```python
from build123d import *

# Parameters (mm, degrees)
BOSS_EXTRUDE1_DEPTH      = 3.302
BOSS_EXTRUDE1_DEPTH_BACK = 17.018
SKETCH2_W                = 11.43
SKETCH2_H                = 12.7
SKETCH2_5_W              = 5.136925293
SKETCH2_5_H              = 12.7
SKETCH2_5_R              = 1.905
BOSS_EXTRUDE2_DEPTH      = 2.54
BOSS_EXTRUDE3_DEPTH      = 2.54
SKETCH4_R                = 2.286
BOSS_EXTRUDE4_DEPTH      = 5.08


with BuildPart() as part:
    # Sketch2 → Boss-Extrude1 (new, two sides: drawn at the far end of the back side and taken through both)
    with BuildSketch(Plane.XY.offset(-BOSS_EXTRUDE1_DEPTH_BACK)):
        with Locations((-75.585738581, 60.932338755)):
            Rectangle(SKETCH2_W, SKETCH2_H)
        with Locations((-87.015738581, 60.932338755)):
            Rectangle(SKETCH2_W, SKETCH2_H)
    extrude(amount=BOSS_EXTRUDE1_DEPTH + BOSS_EXTRUDE1_DEPTH_BACK)

    # Sketch2_5 → Boss-Extrude2 (add)
    # profile 1 of 2: a face of its own
    with BuildSketch(Plane.XY):
        with Locations((-67.302275935, 60.932338755)):
            Rectangle(SKETCH2_5_W, SKETCH2_5_H)
        with Locations((-67.120738581, 60.932338755)):
            Circle(SKETCH2_5_R, mode=Mode.SUBTRACT)
    # profile 2 of 2: a face of its own
    with BuildSketch(Plane.XY):
        with Locations((-95.299201228, 60.932338755)):
            Rectangle(SKETCH2_5_W, SKETCH2_5_H)
        with Locations((-95.480738581, 60.932338755)):
            Circle(SKETCH2_5_R, mode=Mode.SUBTRACT)
    extrude(amount=-BOSS_EXTRUDE2_DEPTH)

    # Sketch3 → Boss-Extrude3 (add)
    with BuildSketch(Plane.XY.offset(3.302)):
        with BuildLine():
            ThreePointArc((-81.923038581, 63.525721047), (-92.730738581, 60.932338755), (-81.923038581, 58.338956464))
            ThreePointArc((-81.923038581, 58.338956464), (-78.633738581, 60.932338755), (-81.923038581, 63.525721047))
        make_face()
    extrude(amount=BOSS_EXTRUDE3_DEPTH)

    # Sketch4 → Boss-Extrude4 (add)
    with BuildSketch(Plane.XY.offset(5.842)):
        with Locations((-87.015738581, 60.932338755)):
            Circle(SKETCH4_R)
    extrude(amount=BOSS_EXTRUDE4_DEPTH)


solid = part.part
```
Here's how the part is built. I have some questions about the finished solid (model axes, mm). A direction names the side the tool comes from. Round coordinates to 2 decimals unless told otherwise and drop trailing zeros. Order: outer loops, then holes, each group sorted by start corner. A loop starts at its lowest first (then second) coordinate and runs counter-clockwise, first axis right, second up. Notation, with made-up numbers: M 11.25,-22 L 53.25,-22 A23 ccw 53.25,5 Z; hole C -28,-4.75 d8. An arc over 180 degrees is marked long. Answer in a Markdown table with one row per item.
Item 1: For faces 1 (the face through (-92.731, 61, -10)), 2 (the face through (-92.731, 61, 2)), 3 (the face through (-69, 62, -2.54)), 4 (the face through (-92.727, 61.146, 4.554)), 5 (the face through (-69, 62, 0)), which set-ups out of +Z, -Z, +X, -X, +Y, -Y let a thin tool reach every point of the face, with its end or its side?
A:
| item | result |
|---|---|
| face 1 | -Z, -X, +Y, -Y |
| face 2 | +Z, -X, +Y, -Y |
| face 3 | -Z, +X, +Y, -Y |
| face 4 | +Z |
| face 5 | +Z, +X, +Y, -Y |
Item 2: I'm going to push flat-ended pins straight in: pin 1 (5.5 mm diameter, centred on x = -82, y = 60, fed in from +Z); pin 2 (2.5 mm diameter, centred on y = 59, z = 2.5, fed in from -X); pin 3 (5.5 mm diameter, centred on x = -67.5, y = 60.5, fed in from +Z); pin 4 (3 mm diameter, centred on x = -67.12, y = 60.93, fed in from -Z). Where does each tip first touch, or does it pass through?
A:
| item | result |
|---|---|
| pin 1 | stops at z = 5.84 |
| pin 2 | stops at x = -92.73 |
| pin 3 | stops at z = 3.3 |
| pin 4 | passes through |
Item 3: Imagine slicing it at D-D, the plane y = 64.5. Write out the boundary of the cut face in (x, z).
A:
| item | result |
|---|---|
| outline | M -97.87,-2.54 L -92.73,-2.54 L -92.73,-17.02 L -69.87,-17.02 L -69.87,-2.54 L -64.73,-2.54 L -64.73,0 L -69.87,0 L -69.87,3.3 L -82.55,3.3 L -82.55,5.84 L -91.48,5.84 L -91.48,3.3 L -92.73,3.3 L -92.73,0 L -97.87,0 Z |
Item 4: Imagine slicing it at B-B, the plane x = -81. Write out the boundary of the cut face in (y, z), and give its area (3 significant figures).
A:
| item | result |
|---|---|
| outline | M 54.58,-17.02 L 67.28,-17.02 L 67.28,3.3 L 63.58,3.3 L 63.58,5.84 L 58.28,5.84 L 58.28,3.3 L 54.58,3.3 Z |
| area | 272 mm2 |
Item 5: Imagine slicing it at C-C, the plane z = -11.5. Write out the boundary of the cut face in (x, y), and give its area (3 significant figures).
A:
| item | result |
|---|---|
| outline | M -92.73,54.58 L -69.87,54.58 L -69.87,67.28 L -92.73,67.28 Z |
| area | 290 mm2 |
Item 6: Thinking about a two-plate mould opening in X: for faces 6 (the face through (-76, 61, 3.302)), 7 (the face through (-69.871, 61, 2)), 8 (the face through (-93.72, 60.2, -1.25)), which applies, +X half, -X half, draft (parallel to the pull), parting line (faces both ways), or undercut?
A:
| item | result |
|---|---|
| face 6 | draft |
| face 7 | +X half |
| face 8 | undercut |
Item 7: If I drill on L1, parallel to X at y = 57, z = 1; L2, parallel to Z at x = -96, y = 64.5; L3, parallel to Z at x = -92.5, y = 62, over which ranges is the centre line in solid material (lowest first)? Write a range as from..to.
A:
| item | result |
|---|---|
| L1 | x = -92.73..-69.87 |
| L2 | z = -2.54..0 |
| L3 | z = -17.02..5.84 |
Item 8: Imagine slicing it at A-A, the plane x = -67. Write out the boundary of the cut face in (y, z).
A:
| item | result |
|---|---|
| outline | M 54.58,-2.54 L 59.03,-2.54 L 59.03,0 L 54.58,0 Z; M 62.83,-2.54 L 67.28,-2.54 L 67.28,0 L 62.83,0 Z |
